Autodesk Inventor part; units mm, degrees
ref_plane "YZ Plane" through (0, 0, 0) normal (1, 0, 0) x (0, 1, 0)
ref_plane "XZ Plane" through (0, 0, 0) normal (0, 1, 0) x (-1, 0, 0)
ref_plane "XY Plane" through (0, 0, 0) normal (0, 0, 1) x (1, 0, 0)
sketch "Эскиз1" plane through (0, 0, 0) normal (0, 1, 0) x (-1, 0, 0)
  arc A0 (40.3387, -155.9498) -> (43.3926, -135.6785) centre (41.8656, -145.8142) ccw
  line L0 (111.6413, -108.8142) -> (38.7953, -108.8142) construction
  line L1 (76.8656, 21.9817) -> (76.8656, -112.0617)
  circle A1 centre (48.8156, -8.8142) radius 3.05
  circle A2 centre (57.9156, -33.8142) radius 3.05
  circle A3 centre (48.8156, -58.8142) radius 3.05
  circle A4 centre (57.9156, -83.8142) radius 3.05
  circle A5 centre (95.8156, -83.8142) radius 3.05
  circle A6 centre (104.9156, -58.8142) radius 3.05
  circle A7 centre (95.8156, -33.8142) radius 3.05
  circle A8 centre (104.9156, -8.8142) radius 3.05
  arc A9 (53.0155, -4.3903) -> (42.8334, -7.6214) centre (48.8156, -8.8142) ccw
  arc A10 (109.3395, -13.0141) -> (100.7157, -4.3903) centre (104.9156, -8.8142) ccw
  arc A11 (109.3395, -63.0141) -> (109.3395, -54.6142) centre (104.9156, -58.8142) ccw
  line L2 (107.9656, -102.3962) -> (107.9656, -66.4566)
  line L3 (107.9656, -51.1717) -> (107.9656, -16.4566)
  line L4 (97.2731, -5.7642) -> (56.4581, -5.7642)
  line L5 (28.3919, -80.0515) -> (42.8334, -7.6214)
  circle A12 centre (41.8656, -145.8142) radius 18 construction
  line L6 (101.8656, -108.8142) -> (101.8656, -72.3334) construction
  line L7 (101.8656, -108.8142) -> (33.562, -180.6784) construction
  line L8 (51.8656, -108.8142) -> (51.8656, -72.3334) construction
  line L9 (96.2539, -114.7184) -> (107.9656, -102.3962)
  line L10 (96.2539, -114.7184) -> (99.1818, -117.5012)
  arc A13 (98.953, -120.5879) -> (99.1818, -117.5012) centre (97.804, -118.9509) ccw
  circle A14 centre (41.8656, -145.8142) radius 45.2548 construction
  circle A15 centre (14.9897, -109.4042) radius 5.05
  circle A16 centre (5.4556, -172.69) radius 5.05
  arc A17 (-5.4216, -171.0513) -> (3.8169, -183.5673) centre (5.4556, -172.69) ccw
  line L11 (98.953, -120.5879) -> (87.305, -132.8431)
  arc A18 (109.3395, -63.0141) -> (107.9656, -66.4566) centre (112.9656, -66.4566) ccw
  arc A19 (107.9656, -51.1717) -> (109.3395, -54.6142) centre (112.9656, -51.1717) ccw
  arc A20 (109.3395, -13.0141) -> (107.9656, -16.4566) centre (112.9656, -16.4566) ccw
  arc A21 (97.2731, -5.7642) -> (100.7157, -4.3903) centre (97.2731, -0.7642) ccw
  arc A22 (53.0155, -4.3903) -> (56.4581, -5.7642) centre (56.4581, -0.7642) ccw
  circle A23 centre (68.7415, -182.2241) radius 5.05
  circle A24 centre (78.2756, -118.9383) radius 5.05
  arc A25 (67.1028, -193.1014) -> (79.6187, -183.8628) centre (68.7415, -182.2241) ccw
  arc A26 (11.5934, -98.9416) -> (4.1125, -107.7655) centre (14.9897, -109.4042) ccw
  line L12 (78.2756, -118.9383) -> (78.2756, -108.8142) construction
  line L13 (78.2756, -118.9383) -> (85.6139, -125.913) construction
  line L14 (67.1028, -193.1014) -> (3.8169, -183.5673)
  line L15 (79.6187, -183.8628) -> (87.305, -132.8431)
  arc A27 (82.6506, -129.0308) -> (83.6843, -128.5167) centre (78.2756, -118.9383) ccw
  arc A28 (11.5934, -98.9416) -> (28.3919, -80.0515) centre (3.8745, -75.1631) ccw
  line L16 (43.3926, -135.6785) -> (0.8724, -129.2728)
  line L17 (40.3387, -155.9498) -> (-2.1815, -149.544)
  line L18 (4.1125, -107.7655) -> (0.8724, -129.2728)
  line L19 (-2.1815, -149.544) -> (-5.4216, -171.0513)
  line L20 (33.562, -180.6784) -> (35.8815, -182.8829)
  line L21 (35.8815, -182.8829) -> (31.2963, -187.7071)
  line L22 (33.562, -180.6784) -> (27.4345, -187.1253)
  point P0 (0, 0)
  point P1 (107.9656, -64.0969)
  point P2 (107.9656, -53.5314)
  point P3 (107.9656, -14.0969)
  point P4 (99.6329, -5.7642)
  point P5 (54.0984, -5.7642)
  point P6 (100.603, -118.8519)
  point P7 (21.7907, -113.1589)
  point P8 (80.5833, -139.9152)
  point P9 (85.6933, -134.5388)
  dimension "d4" = 37.9
  dimension "d5" = 56.1
  dimension "d6" = 6.1
  dimension "d7" = 50
  dimension "d8" = 50
  dimension "d9" = 25
  dimension "d10" = 50
  dimension "d11" = 37.9
  dimension "d12" = 56.1
  dimension "d15" = 35
  dimension "d16" = 37
  dimension "d17" = 20.5
  dimension "d20" = 12.2
  dimension "d21" = 12.2
  dimension "d24" = 3.05
  dimension "d26" = 36
  dimension "d29" = 50
  dimension "d33" = 10.1
  dimension "d36" = 360
  dimension "d38" = 64
  dimension "d44" = 22
  dimension "d45" = 6
  dimension "d49" = 17
  dimension "d52" = 5
  dimension "d54" = 25
  dimension "d55" = 3.2
  dimension "d56" = 91
extrude "Выдавливание1" add sketch "Эскиз1" along normal blind 3 contours A0 L16 L18 A26 A28 L5 A9 A22 L4 A21 A10 A20 L3 A19 A11 A18 L2 L9 L10 A13 L11 L15 A25 L14 L21 L20 L22 A17 L19 L17
sketch "Эскиз2" plane through (0, 3, 0) normal (0, 1, 0) x (1, 0, 0)
  line L0 (-107.9656, 102.3962) -> (-107.9656, 66.4566)
  arc A0 (-109.3395, 63.0141) -> (-109.3395, 54.6142) centre (-104.9156, 58.8142) ccw
  line L1 (-107.9656, 51.1717) -> (-107.9656, 16.4566)
  arc A1 (-109.3395, 13.0141) -> (-100.7157, 4.3903) centre (-104.9156, 8.8142) ccw
  line L2 (-97.2731, 5.7642) -> (-56.4581, 5.7642)
  arc A2 (-53.0155, 4.3903) -> (-42.8334, 7.6214) centre (-48.8156, 8.8142) ccw
  line L3 (-42.8334, 7.6214) -> (-28.3919, 80.0515)
  arc A3 (5.4216, 171.0513) -> (-3.8169, 183.5673) centre (-5.4556, 172.69) ccw
  line L4 (-87.305, 132.8431) -> (-98.953, 120.5879)
  arc A4 (-98.953, 120.5879) -> (-99.1818, 117.5012) centre (-97.804, 118.9509) ccw
  line L5 (-99.1818, 117.5012) -> (-96.2539, 114.7184)
  line L6 (-96.2539, 114.7184) -> (-107.9656, 102.3962)
  circle A5 centre (-95.8156, 33.8142) radius 3.05
  circle A6 centre (-95.8156, 83.8142) radius 3.05
  circle A7 centre (-57.9156, 83.8142) radius 3.05
  circle A8 centre (-48.8156, 58.8142) radius 3.05
  circle A9 centre (-57.9156, 33.8142) radius 3.05
  arc A10 (-40.3387, 155.9498) -> (-43.3926, 135.6785) centre (-41.8656, 145.8142) ccw
  circle A11 centre (-5.4556, 172.69) radius 5.05
  circle A12 centre (-14.9897, 109.4042) radius 5.05
  circle A13 centre (-104.9156, 8.8142) radius 3.05
  circle A14 centre (-104.9156, 58.8142) radius 3.05
  circle A15 centre (-48.8156, 8.8142) radius 3.05
  arc A16 (-109.3395, 63.0141) -> (-107.9656, 66.4566) centre (-112.9656, 66.4566) ccw
  arc A17 (-107.9656, 51.1717) -> (-109.3395, 54.6142) centre (-112.9656, 51.1717) ccw
  arc A18 (-109.3395, 13.0141) -> (-107.9656, 16.4566) centre (-112.9656, 16.4566) ccw
  arc A19 (-97.2731, 5.7642) -> (-100.7157, 4.3903) centre (-97.2731, 0.7642) ccw
  arc A20 (-53.0155, 4.3903) -> (-56.4581, 5.7642) centre (-56.4581, 0.7642) ccw
  arc A21 (-11.5934, 98.9416) -> (-28.3919, 80.0515) centre (-3.8745, 75.1631) ccw
  arc A22 (-11.5934, 98.9416) -> (-4.1125, 107.7655) centre (-14.9897, 109.4042) ccw
  line L7 (-4.1125, 107.7655) -> (-0.8724, 129.2728)
  line L8 (-0.8724, 129.2728) -> (-43.3926, 135.6785)
  line L9 (-40.3387, 155.9498) -> (2.1815, 149.544)
  line L10 (2.1815, 149.544) -> (5.4216, 171.0513)
  line L11 (-3.8169, 183.5673) -> (-27.4345, 187.1253)
  arc A23 (-67.1028, 193.1014) -> (-79.6187, 183.8628) centre (-68.7415, 182.2241) ccw
  line L12 (-79.6187, 183.8628) -> (-87.305, 132.8431)
  line L13 (-27.4345, 187.1253) -> (-33.562, 180.6784)
  line L14 (-33.562, 180.6784) -> (-35.8815, 182.8829)
  line L15 (-35.8815, 182.8829) -> (-31.2963, 187.7071)
  line L16 (-31.2963, 187.7071) -> (-67.1028, 193.1014)
  point P0 (0, 0)
equation "\"d4\" = -d_main_screw_holes + hight_profile_femur - 2 * thickness_profile_femur"
equation "\"d5\" = hight_profile_femur + d_main_screw_holes"
equation "\"d6\" = d_main_screw_holes"
equation "\"d11\" = -d_main_screw_holes + hight_profile_femur - 2 * thickness_profile_femur"
equation "\"d12\" = hight_profile_femur + d_main_screw_holes"
equation "\"d15\" = width_shaft_shift"
equation "\"d20\" = 2 * d_main_screw_holes"
equation "\"d21\" = 2 * d_main_screw_holes"
equation "\"d24\" = 0.5 * d_main_screw_holes"
equation "\"d29\" = width_profile_femur"
equation "\"d2\" = thickness_steel"
equation "\"tolerance_plazma\" = 0.1"
equation "\"thickness_steel\" = 3"
equation "\"d_main_screw_holes\" = 6.1"
equation "\"thickness_profile_tibea\" = 3"
equation "\"hight_shaft_shift\" = 37"
equation "\"thickness_profile_femur\" = 3"
equation "\"width_profile_femur\" = 50"
equation "\"width_shaft_shift\" = 35"
equation "\"hight_profile_femur\" = 50"
equation "\"width_flattened_surface\" = 12"
properties part number "femur_support_steel" material "Сталь"
Here's how the part is built. I have some questions about the finished solid (model axes, mm). A direction names the side the tool comes from. Coordinates: 2 decimals unless noted, no trailing zeros. Order: outer loops, then holes, each group sorted by start corner. A loop starts at its lowest first (then second) coordinate and runs counter-clockwise, first axis right, second up. Notation, with made-up numbers: M -15,81 L 12,81 A19 ccw 12,100 Z; hole C -35,26.5 d11. An arc over 180 degrees is marked long. Answer as a JSON object with one key per item and string values. Group by question number.
(1) Suppose I cut it at B-B, the plane z = -45. Please give me the cut outline in (x, y).
(2) Which directions (+Z, -Z, +X, -X, +Y, -Y) give clear straight access to the entire face, cutting with the end or side of a thin tool? Please do faces 4 (the face through (-33.62, 1.48, -185.26)), 5 (the face through (-46.88, 1.48, -3.03)).
(3) Suppose I cut it at A-A, the plane y = 1. State how many separate pieces and enclosed holes the cut face has, then the cut area to 3 significant figures.
(4) If we mould it in two halves opening along X, with no side actions, what happens to faces 1 (the face through (-65, 3, -97)), 2 (the face through (-102.03, 1.48, -108.64)), 3 (the face through (-97.223, 1.479, -81.108))? For each: released by +X, released by -X, zero draft, split by the parting line, or undercut.
(5) For pin 1 (1 mm diameter, centred on y = 2, z = -137, fed in from -X); pin 2 (1.5 mm diameter, centred on y = 1, z = -103, fed in from -X), each with a flat end and sliding along its axis, tell me the tip position at first contact or that it passes through.
(6) Suppose I cut it at C-C, the plane z = -144. Please give me the cut outline in (x, y), then the cut area to 3 significant figures.
(7) I need wall thicknesses on probe 1 along Z at (x, y) = (-47, 2.7); probe 2 along X at (y, z) = (0.2, -33); probe 3 along Z at (x, y) = (-55.5, 1.9). Which ranges of each line are inside material? Lowest first, please.
Values found:
{
 "1": {"outline": "M -107.97,0 L -35.38,0 L -35.38,3 L -107.97,3 Z"},
 "2": {"face 4": "+Y, -Y", "face 5": "+Z, +Y, -Y"},
 "3": {"separate pieces": "1", "enclosed holes": "12", "area": "13,400 mm^2"},
 "4": {"face 1": "zero draft", "face 2": "released by -X", "face 3": "undercut"},
 "5": {"pin 1": "stops at x = -86.75", "pin 2": "stops at x = -107.97"},
 "6": {"outline": "M -85.62,0 L -51.95,0 L -51.95,3 L -85.62,3 Z", "area": "101 mm^2"},
 "7": {"probe 1": "z = -190.07 to -154.69, -136.94 to -61.26, -56.36 to -11.26, -6.36 to -2.99", "probe 2": "x = -107.97 to -98.75, -92.88 to -60.85, -54.98 to -37.77", "probe 3": "z = -191.35 to -85.68, -81.95 to -35.68, -31.95 to -5.67"}
}
